Source: CAD feature listing. Evaluate the final solid. Frame: model axes, mm. A direction names the side the tool comes from. Give positions to 0.01 mm unless a question says otherwise; leave off trailing zeros. Order: outer loops, then holes, each group sorted by start corner. A loop starts at its lowest first (then second) coordinate and runs counter-clockwise, first axis right, second up. Notation, with made-up numbers: (-12.75, 84.25) - (22.25, 84.25) arc R20 ccw to (22.25, 93.25) - close; hole circle Ø3 at (60.5, 13). An arc over 180 degrees is marked (long way). Answer as CSV lines item,"result".
```python
from build123d import *

# Parameters (mm, degrees)
SKETCH1_W           = 230
SKETCH1_H           = 66
BOSS_EXTRUDE1_DEPTH = 5
SKETCH2_W           = 10
SKETCH2_H           = 10
BOSS_EXTRUDE2_DEPTH = 10
SKETCH3_R           = 1.5
CUT_EXTRUDE1_DEPTH  = 233.83900017
CUT_EXTRUDE2_DEPTH  = 238.67414668


with BuildPart() as part:
    # Sketch1 → Boss-Extrude1 (new body)
    with BuildSketch(Plane(origin=(0, 0, 0), x_dir=(1, 0, 0), z_dir=(0, 1, 0))):
        with Locations((115, 0)):
            Rectangle(SKETCH1_W, SKETCH1_H)
    extrude(amount=BOSS_EXTRUDE1_DEPTH)

    # Sketch2 → Boss-Extrude2 (add)
    with BuildSketch(Plane(origin=(0, 5, 0), x_dir=(1, 0, 0), z_dir=(0, 1, 0))):
        with Locations((5, -20)):
            Rectangle(SKETCH2_W, SKETCH2_H)
        with Locations((225, -20)):
            Rectangle(SKETCH2_W, SKETCH2_H)
        with Locations((225, 20)):
            Rectangle(SKETCH2_W, SKETCH2_H)
        with Locations((5, 20)):
            Rectangle(SKETCH2_W, SKETCH2_H)
    extrude(amount=BOSS_EXTRUDE2_DEPTH)

    # Sketch3 → Cut-Extrude1 (cut, through all)
    with BuildSketch(Plane(origin=(230, 0, 0), x_dir=(0, 0, -1), z_dir=(1, 0, 0))):
        with Locations((-20, 9)):
            Circle(SKETCH3_R)
        with Locations((20, 9)):
            Circle(SKETCH3_R)
    extrude(amount=-CUT_EXTRUDE1_DEPTH, mode=Mode.SUBTRACT)

    # Sketch4 → Cut-Extrude2 (cut, through all)
    with BuildSketch(Plane(origin=(0, 0, -25), x_dir=(-1, 0, 0), z_dir=(0, 0, -1))):
        Polygon((-227.2, 15), (-220, 7.8), (-220, 15), align=None)
        Polygon((-2.8, 15), (-10, 15), (-10, 7.8), align=None)
    extrude(amount=-CUT_EXTRUDE2_DEPTH, mode=Mode.SUBTRACT)


solid = part.part
```
(1) Mould query, pull axis Z, two halves, no side actions, for faces 1 (the flat face through (113, 0, 0)), 2 (the flat face through (226, 9, 15)), 3 (the flat face through (4, 9, -25)). Classes: released by +Z, released by -Z, zero draft, split by the parting line, or undercut.
Completed:
face 1,"zero draft"
face 2,"undercut"
face 3,"released by -Z"
(2) Cut plane A-A (z = 2.5). Return loops of the section in (x, y), then the cut area to 3 significant figures.
Completed:
outline,"(0, 0) - (230, 0) - (230, 5) - (0, 5) - close"
area,"1,150 mm²"
(3) Access query for faces 4 (the flat face through (6.5, 11.3, -20.1)), 5 (the flat face through (226, 9, -25)), 6 (the flat face through (226, 9, 25)), 7 (the flat face through (226, 9, -15)). Directions: +Z, -Z, +X, -X, +Y, -Y. A direction counts if a zero-diameter tool reaches every point of the face in a straight line with its end or side. Return the directions, or none.
Completed:
face 4,"+Z, -Z, +Y"
face 5,"-Z, +X, -X, +Y"
face 6,"+Z, +X, -X, +Y"
face 7,"+X, -X, +Y"
(4) Ray query, line 1 (Z direction, x = 2, y = 9); line 2 (Y direction, x = 227.75, z = -20); line 3 (X direction, y = 5.75, z = 17). Return the intervals inside material, ascending. Write a range as from..to.
Completed:
line 1,"-25..-21.5, -18.5..-15, 15..18.5, 21.5..25"
line 2,"0..7.5, 10.5..15"
line 3,"0..10, 220..230"
(5) Contact query for flat-ended pins moving along their axis: pin 1 (3 mm diameter, centred on x = 196.5, z = -8, fed in from +Y); pin 2 (3 mm diameter, centred on x = 4.5, y = 10, fed in from -Z); pin 3 (3 mm diameter, centred on x = 5, y = 12, fed in from +Z). Output: stop coordinate, or through.
Completed:
pin 1,"y = 5"
pin 2,"z = -25"
pin 3,"z = 25"
(6) Cut plane B-B (x = 41). Return loops of the section in (y, z).
Completed:
outline,"(0, -33) - (5, -33) - (5, 33) - (0, 33) - close"
